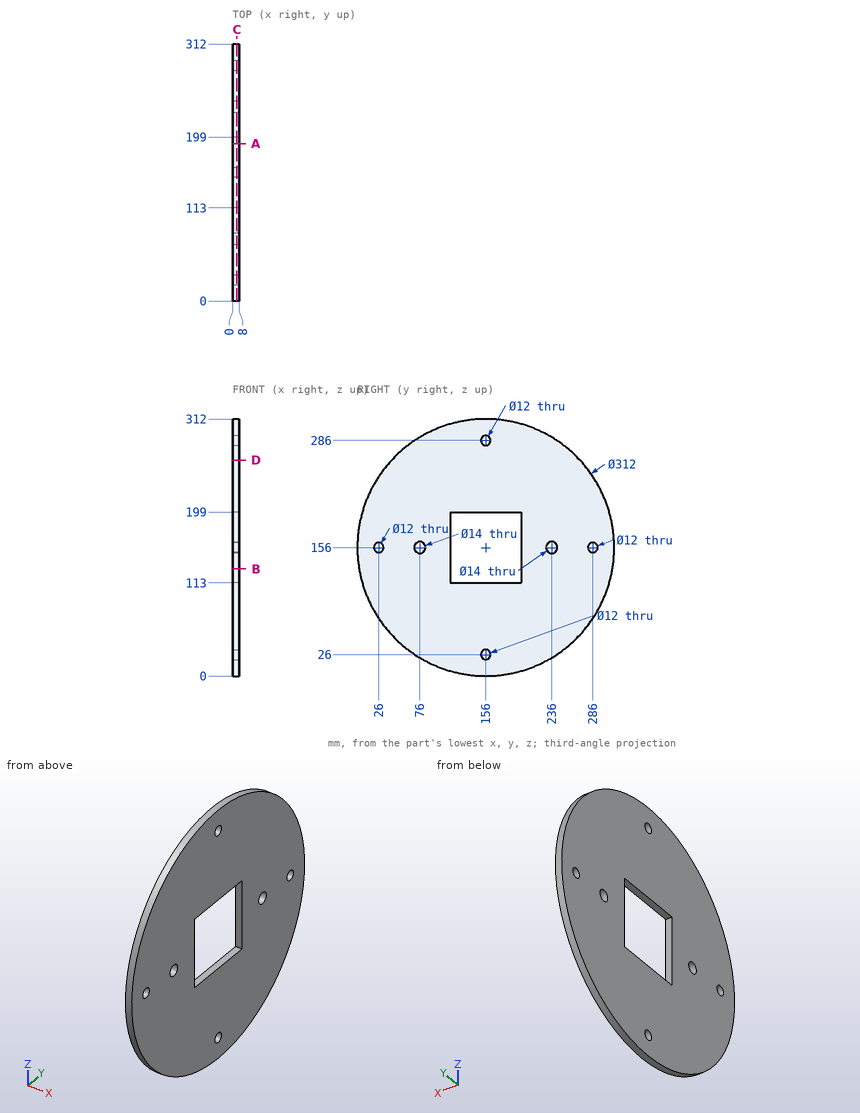
Here's the drawing with two shaded views (mm, measured from the low corner). I have some questions. Coordinates: 2 decimals unless noted, no trailing zeros. Order: outer loops, then holes, each group sorted by start corner. A loop starts at its lowest first (then second) coordinate and runs counter-clockwise, first axis right, second up. Notation, with made-up numbers: (4.5, 80) -> (17.5, 80) arc R14 ccw to (17.5, 86) -> close; hole circle Ø6 at (43, -27). An arc over 180 degrees is marked (long way). One line per question, with ' | ' between items.
Q1. Imagine slicing it at D-D on z = 262. Please give me the cut outline in (x, y), and give its area (3 significant figures).
Return value:
outline: (0, 41.54) -> (8, 41.54) -> (8, 270.46) -> (0, 270.46) -> close | area: 1,830 mm²
Q2. Imagine slicing it at C-C on x = 5. Please give me the cut outline in (y, z).
Return value:
outline: circle Ø312 at (156, 156); hole circle Ø12 at (26, 156); hole circle Ø14 at (76, 156); hole (113, 113) -> (199, 113) -> (199, 199) -> (113, 199) -> close; hole circle Ø12 at (156, 26); hole circle Ø12 at (156, 286); hole circle Ø14 at (236, 156); hole circle Ø12 at (286, 156)
Q3. Imagine slicing it at B-B on z = 130. Please give me the cut outline in (x, y).
Return value:
outline: (0, 2.18) -> (8, 2.18) -> (8, 113) -> (0, 113) -> close; (0, 199) -> (8, 199) -> (8, 309.82) -> (0, 309.82) -> close
Q4. Imagine slicing it at A-A on y = 191. Please give me the cut outline in (x, z), and give its area (3 significant figures).
Return value:
outline: (0, 3.98) -> (8, 3.98) -> (8, 113) -> (0, 113) -> close; (0, 199) -> (8, 199) -> (8, 308.02) -> (0, 308.02) -> close | area: 1,740 mm²
Q5. I'm going to push flat-ended pins straight in: P1, Ø5, axis at y = 101.5, z = 271.5, coming from the -X side; P2, Ø7, axis at y = 156, z = 26, coming from the +X side; P3, Ø4, axis at x = 4, y = 153.5, coming from the +Z side. Where does each tip first touch, or does it pass through?
Return value:
P1: x = 0 | P2: through | P3: z = 312
Q6. If I drill on L1, parallel to Y at x = 5.5, z = 156; L2, parallel to Y at x = 0.5, z = 144; L3, parallel to Y at x = 3, z = 286, over which ranges is the centre line in solid material (lowest first)?
Return value:
L1: 0 to 20, 32 to 69, 83 to 113, 199 to 229, 243 to 280, 292 to 312 | L2: 0.46 to 113, 199 to 311.54 | L3: 69.77 to 150, 162 to 242.23
